CAD build for the part. Positions are in the model's coordinates, mm. A direction names the side the tool comes from. Give positions to 0.01 mm unless a question says otherwise; leave off trailing zeros. Order: outer loops, then holes, each group sorted by start corner. A loop starts at its lowest first (then second) coordinate and runs counter-clockwise, first axis right, second up.
from build123d import *

# Parameters (mm, degrees)
SKETCH_1_W          = 30
SKETCH_1_H          = 95
EXTRUDE_1_DEPTH     = 48
SKETCH_2_R          = 3.025
SKETCH_2_R_2        = 3.005
CUT_EXTRUDE_1_DEPTH = 46
SKETCH_3_W          = 30
SKETCH_3_H          = 20
EXTRUDE_2_DEPTH     = 30
SKETCH_4_R          = 2
CUT_EXTRUDE_2_DEPTH = 5
SKETCH_5_W          = 48
SKETCH_5_H          = 35
CUT_EXTRUDE_3_DEPTH = 127.526677029
SKETCH_6_R          = 2
CUT_EXTRUDE_4_DEPTH = 5


with BuildPart() as part:
    # 草图1 → 凸台-拉伸1 (new body)
    with BuildSketch(Plane.XY):
        with Locations((15, 47.5)):
            Rectangle(SKETCH_1_W, SKETCH_1_H)
    extrude(amount=EXTRUDE_1_DEPTH)

    # 草图2 → 切除-拉伸1 (cut)
    # profile 1 of 2: a face of its own
    with BuildSketch(Plane.ZY):
        with Locations((7, 35)):
            Circle(SKETCH_2_R)
        with Locations((7, 35)):
            Circle(SKETCH_2_R_2, mode=Mode.SUBTRACT)
    # profile 2 of 2: a face of its own
    with BuildSketch(Plane.ZY):
        with Locations((41, 35)):
            Circle(SKETCH_2_R)
        with Locations((41, 35)):
            Circle(SKETCH_2_R_2, mode=Mode.SUBTRACT)
    extrude(amount=-CUT_EXTRUDE_1_DEPTH, mode=Mode.SUBTRACT)


with BuildPart() as cut_extrude_1_kept_piece:
    # of the separate pieces the step leaves, the one the design keeps (cut_extrude_1_pieces_kept)
    add(part.part.solids().sort_by_distance((0, 0, 0))[0])

    # 草图3 → 凸台-拉伸2 (add)
    with BuildSketch(Plane.XY.offset(48)):
        with Locations((15, 85)):
            Rectangle(SKETCH_3_W, SKETCH_3_H)
    extrude(amount=EXTRUDE_2_DEPTH)

    # 草图4 → 切除-拉伸2 (cut)
    with BuildSketch(Plane(origin=(0, 95, 0), x_dir=(1, 0, 0), z_dir=(0, 1, 0))):
        with Locations(Location((5, -72.983651548, 0), (0, 0, 270))):
            Circle(SKETCH_4_R)
        with Locations(Location((15, -72.983651548, 0), (0, 0, 270))):
            Circle(SKETCH_4_R)
        with Locations(Location((25, -72.983651548, 0), (0, 0, 270))):
            Circle(SKETCH_4_R)
    extrude(amount=-CUT_EXTRUDE_2_DEPTH, mode=Mode.SUBTRACT)

    # 草图5 → 切除-拉伸3 (cut, through all)
    with BuildSketch(Plane.ZY):
        with Locations((24, 17.5)):
            Rectangle(SKETCH_5_W, SKETCH_5_H)
    extrude(amount=-CUT_EXTRUDE_3_DEPTH, mode=Mode.SUBTRACT)

    # 草图6 → 切除-拉伸4 (cut)
    with BuildSketch(Plane.XZ.offset(-35)):
        with Locations(Location((6, 31.975, 0), (0, 0, 270))):
            Circle(SKETCH_6_R)
        with Locations(Location((12, 31.975, 0), (0, 0, 270))):
            Circle(SKETCH_6_R)
        with Locations(Location((18, 31.975, 0), (0, 0, 270))):
            Circle(SKETCH_6_R)
        with Locations(Location((24, 31.975, 0), (0, 0, 270))):
            Circle(SKETCH_6_R)
        with Locations(Location((6, 16.025, 0), (0, 0, 270))):
            Circle(SKETCH_6_R)
        with Locations(Location((12, 16.025, 0), (0, 0, 270))):
            Circle(SKETCH_6_R)
        with Locations(Location((18, 16.025, 0), (0, 0, 270))):
            Circle(SKETCH_6_R)
        with Locations(Location((24, 16.025, 0), (0, 0, 270))):
            Circle(SKETCH_6_R)
    extrude(amount=-CUT_EXTRUDE_4_DEPTH, mode=Mode.SUBTRACT)


solid = cut_extrude_1_kept_piece.part
1. Saw through at A-A on x = 12. Give the cut face in (y, z) (3 decimals), plus the area to 3 significant figures.
2. 3-axis set-ups, long thin cutter, end or side, ignore diameter. For faces 4 (the cylindrical face through (12.088, 37.465, 33.973)), 5 (the cylindrical face through (5.6, 92.54, 74.89)), 6 (the cylindrical face through (14.79, 38.024, 41.067)), 7 (the flat face through (15, 35, 24)), 8 (the flat face through (15, 55, 48)): which of +Z, -Z, +X, -X, +Y, -Y reach the whole face in a straight line?
3. Mould opens along X. For faces 1 (the flat face through (15, 75, 63)), 2 (the flat face through (25, 90, 73)), 3 (the flat face through (0, 65, 30)) say: released by +X, released by -X, zero draft, split by the parting line, or undercut.
4. Wall check: line 1 (Z direction, x = 6.5, y = 43); line 2 (Y direction, x = 18.25, z = 15); line 3 (Y direction, x = 25.75, z = 59). Give the ranges that are in metal, low to high.
5. Saw through at D-D on x = 6. Give the cut face in (y, z) (3 decimals).
6. Saw through at B-B on z = 51. Give the cut face in (x, y).
7. Pin check, flat tips, straight feed: P1, Ø6.5, axis at x = 25, z = 72.98, coming from the -Y side; P2, Ø1, axis at x = 15, y = 46.5, coming from the +Z side; P3, Ø4.5, axis at x = 25.5, z = 72, coming from the +Y side; P4, Ø3.5, axis at x = 24, z = 31.975, coming from the -Y side. Stop position of each tip, or through.
8. Saw through at C-C on y = 60. Give the cut face in (x, z), plus the area to 3 significant figures.
Reported:
1. outline: (35, 0) - (95, 0) - (95, 78) - (75, 78) - (75, 48) - (35, 48) - (35, 44.025) arc R3.025 cw to (35, 37.975) - (35, 33.975) - (40, 33.975) - (40, 29.975) - (35, 29.975) - (35, 18.025) - (40, 18.025) - (40, 14.025) - (35, 14.025) - (35, 10.025) arc R3.025 cw to (35, 3.975) - close
1. area: 3,410 mm2
2. face 4: -Y
2. face 5: +Y
2. face 6: +X, -X, -Y
2. face 7: +Z, -Z, +X, -X, -Y
2. face 8: +Z, +X, -X, -Y
3. face 1: zero draft
3. face 2: undercut
3. face 3: released by -X
4. line 1: z = 0 to 48
4. line 2: y = 40 to 95
4. line 3: y = 75 to 95
5. outline: (35, 0) - (95, 0) - (95, 71.252) - (90, 71.252) - (90, 74.716) - (95, 74.716) - (95, 78) - (75, 78) - (75, 48) - (35, 48) - (35, 44.025) arc R3.025 cw to (35, 37.975) - (35, 33.975) - (40, 33.975) - (40, 29.975) - (35, 29.975) - (35, 18.025) - (40, 18.025) - (40, 14.025) - (35, 14.025) - (35, 10.025) arc R3.025 cw to (35, 3.975) - close
6. outline: (0, 75) - (30, 75) - (30, 95) - (0, 95) - close
7. P1: stops at y = 75
7. P2: stops at z = 48
7. P3: stops at y = 95
7. P4: stops at y = 40
8. outline: (0, 0) - (30, 0) - (30, 48) - (0, 48) - close
8. area: 1,440 mm2
